Design review of the part shown in the three views and the two pictorial views. Dimensions are in mm from the part's minimum x, y and z. Coordinates: 2 decimals unless noted, no trailing zeros. Loops run counter-clockwise (first coordinate to the right, second up) from the corner with the lowest first, then second, coordinate; pieces in that order, holes last. Notation, with made-up numbers: (21.25, 13) - (76.25, 13) arc R26 cw to (76.25, 30) - close; hole circle Ø5 at (66, 11). An arc over 180 degrees is marked (long way). One line per question, with ' | ' between items.
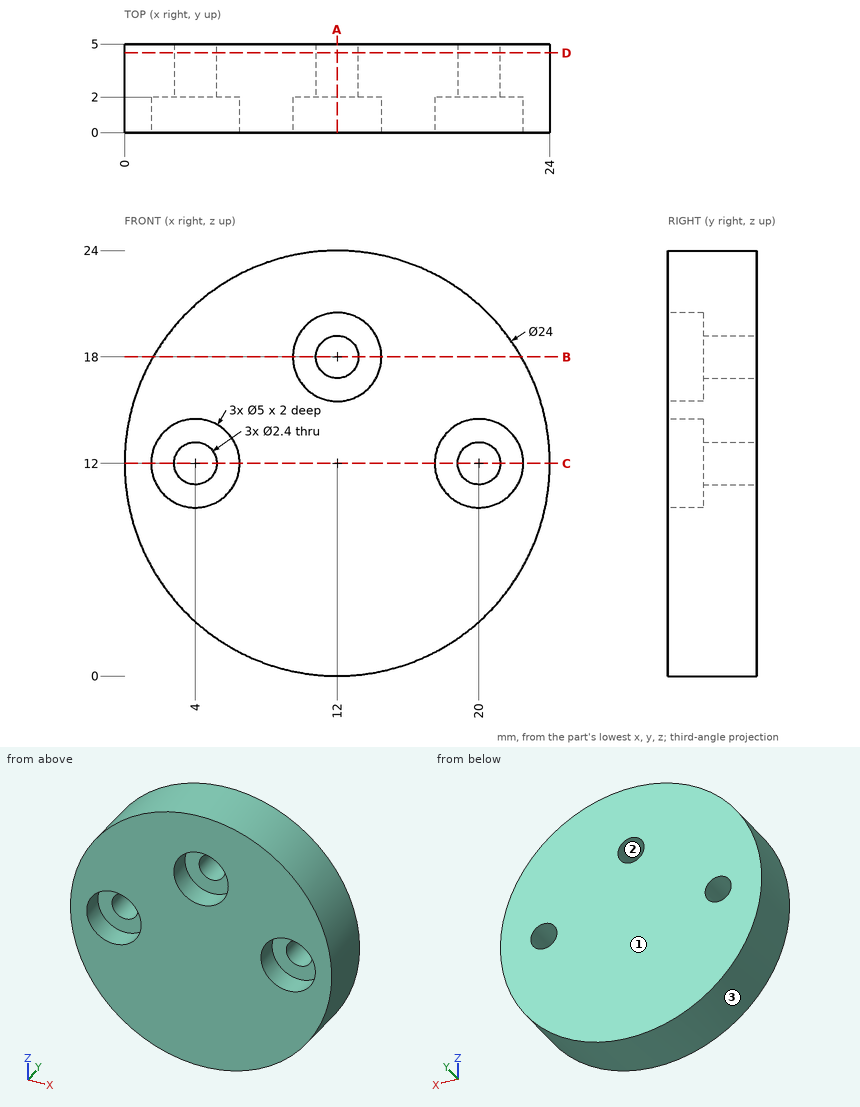
Q1. For pin 1 (1.5 mm diameter, centred on x = 21, z = 12.5, fed in from -Y); pin 2 (5.5 mm diameter, centred on x = 3.5, z = 12, fed in from -Y); pin 3 (1.4 mm diameter, centred on x = 4, z = 12, fed in from -Y); pin 4 (1 mm diameter, centred on y = 4, z = 13.5, fed in from -X), all flat-tipped, find the tip position at first contact; note any pin that passes through.
Returned:
pin 1: stops at y = 2 | pin 2: stops at y = 0 | pin 3: passes through | pin 4: stops at x = 0.04
Q2. To check wall thickness, follow line 1 along Z through (x, y) = (12, 1.4); line 2 along X through (y, z) = (1.6, 11.25); line 3 along Z through (x, y) = (4, 2.5). State the ranges of each line that lie inside material, in increasing order.
Returned:
line 1: z = 0 to 15.5, 20.5 to 24 | line 2: x = 0.02 to 1.62, 6.38 to 17.62, 22.38 to 23.98 | line 3: z = 3.06 to 10.8, 13.2 to 20.94
Q3. Take a section at A-A (x = 12). Give the boundary of the cut face in (y, z), plus the area to 3 significant figures.
Returned:
outline: (0, 0) - (5, 0) - (5, 16.8) - (2, 16.8) - (2, 15.5) - (0, 15.5) - close; (0, 20.5) - (2, 20.5) - (2, 19.2) - (5, 19.2) - (5, 24) - (0, 24) - close | area: 103 mm²
Q4. Take a section at D-D (y = 4.5). Give the boundary of the cut face in (x, z), plus the area to 3 significant figures.
Returned:
outline: circle Ø24 at (12, 12); hole circle Ø2.4 at (4, 12); hole circle Ø2.4 at (12, 18); hole circle Ø2.4 at (20, 12) | area: 439 mm²
Q5. Draft analysis for pull direction X (two halves, no side actions). For the marked faces 1, 2 and 3, state which applies: +X half, -X half, draft (parallel to the pull), parting line (faces both ways), or undercut.
Returned:
face 1: draft | face 2: undercut | face 3: parting line
Q6. Take a section at B-B (z = 18). Give the boundary of the cut face in (x, y), plus the area to 3 significant figures.
Returned:
outline: (1.61, 0) - (9.5, 0) - (9.5, 2) - (10.8, 2) - (10.8, 5) - (1.61, 5) - close; (13.2, 2) - (14.5, 2) - (14.5, 0) - (22.39, 0) - (22.39, 5) - (13.2, 5) - close | area: 86.7 mm²
Q7. Take a section at C-C (z = 12). Give the boundary of the cut face in (x, y).
Returned:
outline: (0, 0) - (1.5, 0) - (1.5, 2) - (2.8, 2) - (2.8, 5) - (0, 5) - close; (5.2, 2) - (6.5, 2) - (6.5, 0) - (17.5, 0) - (17.5, 2) - (18.8, 2) - (18.8, 5) - (5.2, 5) - close; (21.2, 2) - (22.5, 2) - (22.5, 0) - (24, 0) - (24, 5) - (21.2, 5) - close
